Source: CAD feature listing. Evaluate the final solid. Frame: model axes, mm. Give positions to 0.01 mm unless a question says otherwise; leave off trailing zeros. Order: outer loops, then holes, each group sorted by start corner. A loop starts at its lowest first (then second) coordinate and runs counter-clockwise, first axis right, second up. Notation, with made-up numbers: (-15.5, 34.5) - (-9.5, 34.5) arc R25 ccw to (-9.5, 63.5) - close; hole circle Ø9 at (6, -20). An arc over 180 degrees is marked (long way). Use CSV: the item, a comma, the result in double quotes.
```python
from build123d import *

# Parameters (mm, degrees)
SKETCH_1_R          = 13.5
SKETCH_1_R_2        = 1.5
EXTRUDE_1_DEPTH     = 4
CUT_EXTRUDE_2_DEPTH = 72.640840308
FILLET_1_R          = 2


with BuildPart() as part:
    # 草图1 → 凸台-拉伸1 (new body)
    with BuildSketch(Plane(origin=(0, 0, 0), x_dir=(1, 0, 0), z_dir=(0, 1, 0))):
        with BuildLine():
            Line((36.9, 42), (-36.9, 42))
            ThreePointArc((-36.9, 42), (-57.9, 21), (-36.9, 0))
            Line((-36.9, 0), (36.9, 0))
            ThreePointArc((36.9, 0), (57.9, 21), (36.9, 42))
        make_face()
        with Locations(Location((-36.9, 21, 0), (0, 0, 270))):
            Circle(SKETCH_1_R, mode=Mode.SUBTRACT)
        with Locations(Location((-36.9, 38.5, 0), (0, 0, 270))):
            Circle(SKETCH_1_R_2, mode=Mode.SUBTRACT)
        with Locations(Location((-24.525631329, 33.374368671, 0), (0, 0, 270))):
            Circle(SKETCH_1_R_2, mode=Mode.SUBTRACT)
        with Locations(Location((-19.4, 21, 0), (0, 0, 270))):
            Circle(SKETCH_1_R_2, mode=Mode.SUBTRACT)
        with Locations(Location((-24.525631329, 8.625631329, 0), (0, 0, 270))):
            Circle(SKETCH_1_R_2, mode=Mode.SUBTRACT)
        with Locations(Location((-36.9, 3.5, 0), (0, 0, 270))):
            Circle(SKETCH_1_R_2, mode=Mode.SUBTRACT)
        with Locations(Location((-49.274368671, 8.625631329, 0), (0, 0, 270))):
            Circle(SKETCH_1_R_2, mode=Mode.SUBTRACT)
        with Locations(Location((-54.4, 21, 0), (0, 0, 270))):
            Circle(SKETCH_1_R_2, mode=Mode.SUBTRACT)
        with Locations(Location((-49.274368671, 33.374368671, 0), (0, 0, 270))):
            Circle(SKETCH_1_R_2, mode=Mode.SUBTRACT)
        with Locations(Location((49.274368671, 33.374368671, 0), (0, 0, 90))):
            Circle(SKETCH_1_R_2, mode=Mode.SUBTRACT)
        with Locations(Location((54.4, 21, 0), (0, 0, 90))):
            Circle(SKETCH_1_R_2, mode=Mode.SUBTRACT)
        with Locations(Location((49.274368671, 8.625631329, 0), (0, 0, 90))):
            Circle(SKETCH_1_R_2, mode=Mode.SUBTRACT)
        with Locations(Location((36.9, 3.5, 0), (0, 0, 90))):
            Circle(SKETCH_1_R_2, mode=Mode.SUBTRACT)
        with Locations(Location((24.525631329, 8.625631329, 0), (0, 0, 90))):
            Circle(SKETCH_1_R_2, mode=Mode.SUBTRACT)
        with Locations(Location((19.4, 21, 0), (0, 0, 90))):
            Circle(SKETCH_1_R_2, mode=Mode.SUBTRACT)
        with Locations(Location((24.525631329, 33.374368671, 0), (0, 0, 90))):
            Circle(SKETCH_1_R_2, mode=Mode.SUBTRACT)
        with Locations(Location((36.9, 38.5, 0), (0, 0, 90))):
            Circle(SKETCH_1_R_2, mode=Mode.SUBTRACT)
        with Locations(Location((36.9, 21, 0), (0, 0, 90))):
            Circle(SKETCH_1_R, mode=Mode.SUBTRACT)
    extrude(amount=EXTRUDE_1_DEPTH)

    # 草图2 → 切除-拉伸2 (cut, through all)
    with BuildSketch(Plane(origin=(0, 0, 0), x_dir=(1, 0, 0), z_dir=(0, 1, 0))):
        Polygon((21.358748179, 37), (-21.358748179, 37), (-14.735151519, 23.5), (14.735151519, 23.5), align=None)
        Polygon((21.358748179, 5), (-21.358748179, 5), (-14.735151519, 18.5), (14.735151519, 18.5), align=None)
    extrude(amount=CUT_EXTRUDE_2_DEPTH, mode=Mode.SUBTRACT)

    # 圆角1
    fillet_1_edges = [part.edges().sort_by_distance(p)[0] for p in [
        (-21.358748179, 2, -37),
        (-14.735151519, 2, -23.5),
        (14.735151519, 2, -23.5),
        (21.358748179, 2, -37),
        (21.358748179, 2, -5),
        (14.735151519, 2, -18.5),
        (-14.735151519, 2, -18.5),
        (-21.358748179, 2, -5),
    ]]
    fillet(fillet_1_edges, radius=FILLET_1_R)


solid = part.part
```
Item 1: Section D-D on x = 30.5. Return the cut outline in (y, z).
Filled in:
outline,"(0, -42) - (4, -42) - (4, -32.89) - (0, -32.89) - close; (0, -9.11) - (4, -9.11) - (4, 0) - (0, 0) - close"
Item 2: Mould query, pull axis X, two halves, no side actions, for faces 1 (the cylindrical face through (-52.913, 1.972, -21.195)), 2 (the cylindrical face through (-57.895, 1.972, -21.462)). Classes: released by +X, released by -X, zero draft, split by the parting line, or undercut.
Filled in:
face 1,"undercut"
face 2,"released by -X"
Item 3: Material intervals for line 1 (Z direction, x = 36.9, y = 2.25); line 2 (Z direction, x = -11.5, y = 2.35); line 3 (Z direction, x = -38, y = 1.1), sorted ascending. Write a range as from..to.
Filled in:
line 1,"z = -42..-40, -37..-34.5, -7.5..-5, -2..0"
line 2,"z = -42..-37, -23.5..-18.5, -5..0"
line 3,"z = -41.97..-39.52, -37.48..-34.46, -7.54..-4.52, -2.48..-0.03"
Item 4: Section A-A on x = -2.5. Return the cut outline in (y, z), then the cut area to 3 significant figures.
Filled in:
outline,"(0, -42) - (4, -42) - (4, -37) - (0, -37) - close; (0, -23.5) - (4, -23.5) - (4, -18.5) - (0, -18.5) - close; (0, -5) - (4, -5) - (4, 0) - (0, 0) - close"
area,"60.0 mm2"
Item 5: Section B-B on z = -21. Return the cut outline in (x, y).
Filled in:
outline,"(-57.9, 0) - (-55.9, 0) - (-55.9, 4) - (-57.9, 4) - close; (-52.9, 0) - (-50.4, 0) - (-50.4, 4) - (-52.9, 4) - close; (-23.4, 0) - (-20.9, 0) - (-20.9, 4) - (-23.4, 4) - close; (-17.9, 0) - (17.9, 0) - (17.9, 4) - (-17.9, 4) - close; (20.9, 0) - (23.4, 0) - (23.4, 4) - (20.9, 4) - close; (50.4, 0) - (52.9, 0) - (52.9, 4) - (50.4, 4) - close; (55.9, 0) - (57.9, 0) - (57.9, 4) - (55.9, 4) - close"
Item 6: First-contact query: pin 1 (2.5 mm diameter, centred on x = 49.27, z = -8.63, fed in from +Y); pin 2 (5 mm diameter, centred on x = 54.4, z = -21, fed in from +Y); pin 3 (2 mm diameter, centred on y = 2.5, z = -26, fed in from -X). Flat tips, straight axial feed; report the tip coordinate or a pass-through.
Filled in:
pin 1,"passes through"
pin 2,"stops at y = 4"
pin 3,"stops at x = -57.52"
Item 7: Section C-C on z = -15. Return the cut outline in (x, y).
Filled in:
outline,"(-57.02, 0) - (-48.99, 0) - (-48.99, 4) - (-57.02, 4) - close; (-24.81, 0) - (-16.45, 0) - (-16.45, 4) - (-24.81, 4) - close; (16.45, 0) - (24.81, 0) - (24.81, 4) - (16.45, 4) - close; (48.99, 0) - (57.02, 0) - (57.02, 4) - (48.99, 4) - close"
